Geometry: final body of the model. Coordinates: model frame, mm. Face numbers are marked on the shaded views. A direction names the side the tool comes from. Round coordinates to 2 decimals unless told otherwise and drop trailing zeros. Loops run counter-clockwise (first coordinate to the right, second up) from the corner with the lowest first, then second, coordinate; pieces in that order, holes last. Notation, with made-up numbers: (84.5, 26.25) -> (88.5, 26.25) arc R29 cw to (88.5, 47.25) -> close; hole circle Ø8 at (51, -25). An arc over 180 degrees is marked (long way). Answer in a Markdown table with one row per item.
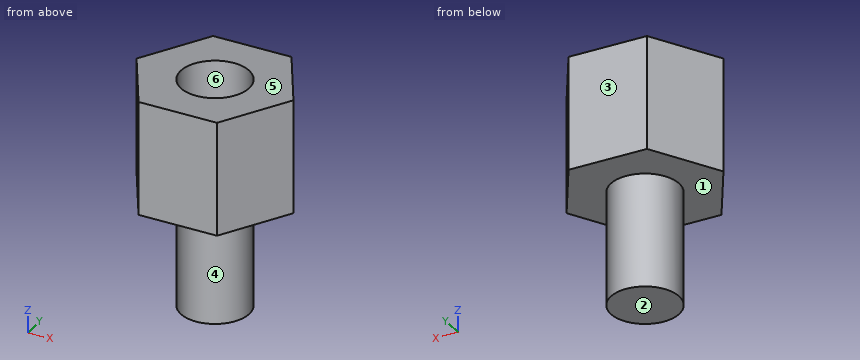
```python
from build123d import *

# Parameters (mm, degrees)
SKETCH_1_R          = 1.5
EXTRUDE_1_DEPTH     = 5
EXTRUDE_2_DEPTH     = 5
SKETCH_3_R          = 1.5
CUT_EXTRUDE_1_DEPTH = 4


with BuildPart() as part:
    # Эскиз1 → Бобышка-Вытянуть1 (new body)
    with BuildSketch(Plane.XY):
        Circle(SKETCH_1_R)
    extrude(amount=EXTRUDE_1_DEPTH)

    # Эскиз2 → Бобышка-Вытянуть2 (add)
    with BuildSketch(Plane.XY.offset(5)):
        Polygon((-3.464101615, 0), (-1.732050808, -3), (1.732050808, -3), (3.464101615, 0), (1.732050808, 3), (-1.732050808, 3), align=None)
    extrude(amount=EXTRUDE_2_DEPTH)

    # Эскиз3 → Вырез-Вытянуть1 (cut)
    with BuildSketch(Plane.XY.offset(10)):
        Circle(SKETCH_3_R)
    extrude(amount=-CUT_EXTRUDE_1_DEPTH, mode=Mode.SUBTRACT)


solid = part.part
```
Item 1: Draft query along Y for the marked faces 3, 4, 5 and 6. Return one class per face: pulls with the +Y half, pulls with the -Y half, needs draft (parallel to the pull), parting line crosses it, or undercut.
Answer:
| item | result |
|---|---|
| face 3 | pulls with the +Y half |
| face 4 | parting line crosses it |
| face 5 | needs draft |
| face 6 | undercut |
Item 2: Line query: probe 1 along Y at (x, z) = (0, 8.85); probe 2 along Z at (x, y) = (-2.5, -1); probe 3 along Z at (x, y) = (-0.5, 1.25). Output: solid intervals per line, ascending. Write a range as [from, to].
Answer:
| item | result |
|---|---|
| probe 1 | y = [-3, -1.5], [1.5, 3] |
| probe 2 | z = [5, 10] |
| probe 3 | z = [0, 6] |
Item 3: Cut plane C-C (z = 5.25). Output: boundary loops of the cut face in (x, y).
Answer:
| item | result |
|---|---|
| outline | (-3.46, 0) -> (-1.73, -3) -> (1.73, -3) -> (3.46, 0) -> (1.73, 3) -> (-1.73, 3) -> close |
Item 4: Reachability of the marked faces 1 and 2 from +Z, -Z, +X, -X, +Y, -Y: full face, straight path, thin tool, end or side. Return the list, or none.
Answer:
| item | result |
|---|---|
| face 1 | -Z |
| face 2 | -Z, +X, -X, +Y, -Y |
Item 5: Cut plane D-D (y = 0.5). Output: boundary loops of the cut face in (x, z), then the cut area to 3 significant figures.
Answer:
| item | result |
|---|---|
| outline | (-3.18, 5) -> (-1.41, 5) -> (-1.41, 0) -> (1.41, 0) -> (1.41, 5) -> (3.18, 5) -> (3.18, 10) -> (1.41, 10) -> (1.41, 6) -> (-1.41, 6) -> (-1.41, 10) -> (-3.18, 10) -> close |
| area | 34.6 mm² |
Item 6: Cut plane B-B (x = 0). Output: boundary loops of the cut face in (y, z).
Answer:
| item | result |
|---|---|
| outline | (-3, 5) -> (-1.5, 5) -> (-1.5, 0) -> (1.5, 0) -> (1.5, 5) -> (3, 5) -> (3, 10) -> (1.5, 10) -> (1.5, 6) -> (-1.5, 6) -> (-1.5, 10) -> (-3, 10) -> close |
Item 7: Cut plane A-A (z = 8.25). Output: boundary loops of the cut face in (x, y), then the cut area to 3 significant figures.
Answer:
| item | result |
|---|---|
| outline | (-3.46, 0) -> (-1.73, -3) -> (1.73, -3) -> (3.46, 0) -> (1.73, 3) -> (-1.73, 3) -> close; hole circle Ø3 at (0, 0) |
| area | 24.1 mm² |
